Autodesk Inventor part; units mm, degrees
ref_plane "YZ Plane" through (0, 0, 0) normal (1, 0, 0) x (0, 1, 0)
ref_plane "XZ Plane" through (0, 0, 0) normal (0, 1, 0) x (-1, 0, 0)
ref_plane "XY Plane" through (0, 0, 0) normal (0, 0, 1) x (1, 0, 0)
sketch "Sketch1" plane through (0, 0, 0) normal (0, 1, 0) x (-1, 0, 0)
  line L0 (0, 0) -> (-50.8, 0)
  line L1 (-50.8, 0) -> (-50.8, -50.8)
  line L2 (-50.8, -50.8) -> (0, -50.8)
  line L3 (0, -50.8) -> (0, 0)
  circle A0 centre (-6.8961, -8.4053) radius 1.5
  circle A1 centre (-6.8961, -42.4053) radius 1.5
  circle A2 centre (-6.8961, -42.4053) radius 2.5
  circle A3 centre (-6.8961, -8.4053) radius 2.5
  circle A4 centre (-43.8961, -8.3947) radius 1.4986
  circle A5 centre (-43.8961, -42.4053) radius 1.4986
  circle A6 centre (-43.8961, -42.4053) radius 2.5019
  circle A7 centre (-43.8961, -8.3947) radius 2.5019
  dimension "d9" = 50.8
  dimension "d10" = 50.8
  dimension "d11" = 3
  dimension "d12" = 3
  dimension "d13" = 34
  dimension "d14" = 5
  dimension "d15" = 5
  dimension "d16" = 8.3947
  dimension "d17" = 2.9972
  dimension "d18" = 2.9972
  dimension "d19" = 5.0038
  dimension "d20" = 5.0038
  dimension "d21" = 34.0106
  dimension "d22" = 37
  dimension "d23" = 37
  dimension "d24" = 6.8961
extrude "Extrusion1" add sketch "Sketch1" along normal blind 2.54 contours L3 L2 L1 L0
extrude "Extrusion2" add sketch "Sketch1" along normal blind 5.08 contours A2 | A3 | A6 | A7
fillet "Fillet1" radius 3.175 4 edges at (0, 1.27, -50.8) (50.8, 1.27, -50.8) (50.8, 1.27, 0) (0, 1.27, 0)
sketch "Sketch3" plane through (0, 2.54, 0) normal (0, 1, 0) x (1, 0, 0)
  line L0 (25.4, 22.225) -> (31.75, 22.225)
  line L1 (31.75, 22.225) -> (31.75, 28.575)
  line L2 (31.75, 28.575) -> (25.4, 28.575)
  line L3 (25.4, 28.575) -> (25.4, 31.75)
  line L4 (25.4, 31.75) -> (19.05, 25.4)
  line L5 (19.05, 25.4) -> (25.4, 19.05)
  line L6 (25.4, 19.05) -> (25.4, 22.225)
  line L7 (47.625, 50.8) -> (3.175, 50.8)
  line L8 (0, 47.625) -> (0, 3.175)
  point P0 (0, 0)
  point P1 (25.4, 20.6375)
  dimension "d40" = 6.35
  dimension "d41" = 6.35
  dimension "d42" = 6.35
  dimension "d43" = 3.175
  dimension "d44" = 45
  dimension "d45" = 22.225
  dimension "d47" = 6.35
  dimension "d48" = 19.05
extrude "Extrusion4" cut sketch "Sketch3" against normal blind 1.27
properties part number "Pump Jig V1"
Read the model definition and answer for the solid it produces. Units are mm, in the model's axes. A direction names the side the tool comes from. Coordinates: 2 decimals unless noted, no trailing zeros. Loops run counter-clockwise (first coordinate to the right, second up) from the corner with the lowest first, then second, coordinate; pieces in that order, holes last. Notation, with made-up numbers: (-23.5, -1) - (-6.5, -1) arc R18 cw to (-6.5, 17) - close; hole circle Ø7 at (2, -9). An arc over 180 degrees is marked (long way). Answer in a Markdown table with one row per item.
Q1. Find section B-B on z = -20. Write down the section's boundary in (x, y), plus the area to 3 significant figures.
Here are the results:
| item | result |
|---|---|
| outline | (0, 0) - (50.8, 0) - (50.8, 2.54) - (25.4, 2.54) - (25.4, 1.27) - (24.45, 1.27) - (24.45, 2.54) - (0, 2.54) - close |
| area | 128 mm^2 |
Q2. Straight lines are drawn through the part: line 1 along Z through (x, y) = (7, 0.8); line 2 along Y through (x, z) = (21.5, -42); line 3 along Z through (x, y) = (20.5, 1.8). For each, find the intervals that lie inside material, in ascending order. Write a range as [from, to].
Here are the results:
| item | result |
|---|---|
| line 1 | z = [-50.8, -43.9], [-40.91, -9.9], [-6.91, 0] |
| line 2 | y = [0, 2.54] |
| line 3 | z = [-50.8, -26.85], [-23.95, 0] |
Q3. Given P1, Ø1.5, axis at y = 3.5, z = -14.5, coming from the -X side; P2, Ø6, axis at x = 21, z = -34, coming from the +Y side, each flat-ended and moving along its own axis, determine where each tip first touches the part or whether it passes through.
Here are the results:
| item | result |
|---|---|
| P1 | passes through |
| P2 | stops at y = 2.54 |
Q4. Find section D-D on z = -12. Write down the section's boundary in (x, y), plus the area to 3 significant figures.
Here are the results:
| item | result |
|---|---|
| outline | (0, 0) - (50.8, 0) - (50.8, 2.54) - (0, 2.54) - close |
| area | 129 mm^2 |
Q5. Find section A-A on y = 3.2. Write down the section's boundary in (x, z).
Here are the results:
| item | result |
|---|---|
| outline | circle Ø5 at (6.9, -42.41); circle Ø5 at (6.9, -8.41); circle Ø5 at (43.9, -42.41); circle Ø5 at (43.9, -8.39); hole circle Ø3 at (6.9, -42.41); hole circle Ø3 at (6.9, -8.41); hole circle Ø3 at (43.9, -42.41); hole circle Ø3 at (43.9, -8.39) |
Q6. For faces 1 (the cylindrical face through (45.9, 3.8, -6.9)), 2 (the flat face through (5, 5.08, -42)), determine the directions among +Z, -Z, +X, -X, +Y, -Y from which every point of the face is accessible in a straight line to the end or side of a thin tool.
Here are the results:
| item | result |
|---|---|
| face 1 | +Y |
| face 2 | +Z, -Z, +X, -X, +Y |
Q7. Find section C-C on x = 27. Write down the section's boundary in (y, z) (3 decimals), plus the area to 3 significant figures.
Here are the results:
| item | result |
|---|---|
| outline | (0, -50.8) - (2.54, -50.8) - (2.54, -28.575) - (1.27, -28.575) - (1.27, -22.225) - (2.54, -22.225) - (2.54, 0) - (0, 0) - close |
| area | 121 mm^2 |
